Geometry: final body of the model. Coordinates: model frame, mm. Face numbers are marked on the shaded views. A direction names the side the tool comes from. Give positions to 0.01 mm unless a question says otherwise; leave off trailing zeros. Write each loop counter-clockwise with the first axis right and the second up, starting at its lowest first coordinate (ties: lowest second). Pieces come first, ordered by that corner, then holes. Notation, with made-up numbers: M 19,-20 L 29,-20 A11 cw 29,-15 Z; hole C 48,-5 d2. An arc over 180 degrees is marked long. One line per question, with ' | ' between items.
from build123d import *

# Parameters (mm, degrees)
PAD_DEPTH       = 22
SKETCH001_W     = 16
SKETCH001_H     = 16
POCKET_DEPTH    = 39.001
SKETCH002_W     = 38
SKETCH002_H     = 85
POCKET001_DEPTH = 15
SKETCH003_R     = 1.8
POCKET002_DEPTH = 7.001
SKETCH004_R     = 3.6
POCKET003_DEPTH = 3
FILLET_R        = 4
FILLET001_R     = 4
SKETCH005_W     = 87.5
SKETCH005_H     = 3.5
POCKET004_DEPTH = 0.5
SKETCH006_R     = 1.8
POCKET005_DEPTH = 22.001
SKETCH007_R     = 3.6
POCKET006_DEPTH = 3
FILLET002_R     = 4
CHAMFER_SIZE    = 3
SKETCH018_R     = 4.25
POCKET016_DEPTH = 5


with BuildPart() as part:
    # Sketch → Pad (new body)
    with BuildSketch(Plane.XY):
        Polygon((39, 0), (39, 25), (70, 25), (70, 76), (63, 83), (63, 115), (78, 115), (78, 0.241195), align=None)
    extrude(amount=PAD_DEPTH)

    # Sketch001 → Pocket (cut, through all)
    with BuildSketch(Plane.YZ.offset(78)):
        with Locations((7, 15)):
            Rectangle(SKETCH001_W, SKETCH001_H)
        with Locations((108, 15)):
            Rectangle(SKETCH001_W, SKETCH001_H)
    extrude(amount=-POCKET_DEPTH, mode=Mode.SUBTRACT)

    # Sketch002 → Pocket001 (cut)
    with BuildSketch(Plane.XY.offset(22)):
        with Locations((56, 57.5)):
            Rectangle(SKETCH002_W, SKETCH002_H)
    extrude(amount=-POCKET001_DEPTH, mode=Mode.SUBTRACT)

    # Sketch003 → Pocket002 (cut, through all)
    with BuildSketch(Plane.XY.offset(7)):
        with Locations((68, 94.119095)):
            Circle(SKETCH003_R)
        with Locations((44, 20.129047)):
            Circle(SKETCH003_R)
    extrude(amount=-POCKET002_DEPTH, mode=Mode.SUBTRACT)

    # Sketch004 → Pocket003 (cut)
    with BuildSketch(Plane.XY.offset(7)):
        with Locations((68, 94.116013)):
            Circle(SKETCH004_R)
        with Locations((44, 20.124216)):
            Circle(SKETCH004_R)
    extrude(amount=-POCKET003_DEPTH, mode=Mode.SUBTRACT)

    # Fillet
    fillet_edges = [part.edges().sort_by_distance(p)[0] for p in [
        (39, 25, 3.5),
        (70, 25, 3.5),
    ]]
    fillet(fillet_edges, radius=FILLET_R)

    # Fillet001
    fillet001_edges = [part.edges().sort_by_distance(p)[0] for p in [
        (63, 83, 3.5),
        (70, 76, 3.5),
    ]]
    fillet(fillet001_edges, radius=FILLET001_R)

    # Sketch005 → Pocket004 (cut)
    with BuildSketch(Plane.YZ.offset(78)):
        with Locations((57.25, 14.5)):
            Rectangle(SKETCH005_W, SKETCH005_H)
    extrude(amount=-POCKET004_DEPTH, mode=Mode.SUBTRACT)

    # Sketch006 → Pocket005 (cut, through all)
    with BuildSketch(Plane(origin=(0, 0, 0), x_dir=(1, 0, 0), z_dir=(0, 0, -1))):
        with Locations((70, -107.5)):
            Circle(SKETCH006_R)
        with Locations((57.5, -7.5)):
            Circle(SKETCH006_R)
    extrude(amount=-POCKET005_DEPTH, mode=Mode.SUBTRACT)

    # Sketch007 → Pocket006 (cut)
    with BuildSketch(Plane(origin=(0, 0, 0), x_dir=(1, 0, 0), z_dir=(0, 0, -1))):
        with Locations((57.5, -7.5)):
            Circle(SKETCH007_R)
        with Locations((70, -107.5)):
            Circle(SKETCH007_R)
    extrude(amount=-POCKET006_DEPTH, mode=Mode.SUBTRACT)

    # Fillet002
    fillet002_edges = [part.edges().sort_by_distance(p)[0] for p in [
        (39, 0, 3.5),
        (78, 0.241195, 3.5),
        (78, 115, 3.5),
        (63, 115, 3.5),
    ]]
    fillet(fillet002_edges, radius=FILLET002_R)

    # Chamfer
    chamfer_edges = [part.edges().sort_by_distance(p)[0] for p in [
        (75, 57.5, 7),
    ]]
    chamfer(chamfer_edges, length=CHAMFER_SIZE)

    # Sketch018 → Pocket016 (cut, symmetric)
    with BuildSketch(Plane.XY.offset(7)):
        with Locations((44, 20.095486)):
            Circle(SKETCH018_R)
        with Locations((68, 94.107513)):
            Circle(SKETCH018_R)
    extrude(amount=POCKET016_DEPTH, both=True, mode=Mode.SUBTRACT)


solid = part.part
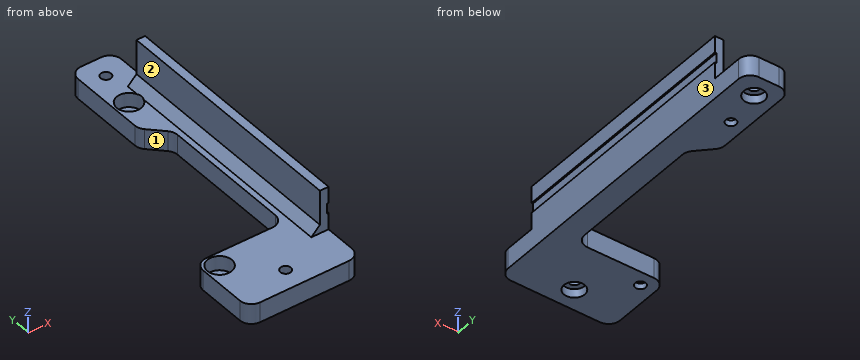
(1) Material intervals for L1, parallel to X at y = 107.5, z = 4.9; L2, parallel to Y at x = 68, z = 1; L3, parallel to Y at x = 44, z = 0.75, sorted ascending. Write a range as [from, to].
Working result:
L1: x = [63, 68.2], [71.8, 78] | L2: y = [0.18, 25.54], [78, 92.32], [95.92, 104.51], [110.49, 115] | L3: y = [0.03, 18.33], [21.93, 25]
(2) Cut plane A-A, the plane y = 7.5. Return loops of the section in (x, z).
Working result:
outline: M 39,0 L 53.9,0 L 53.9,3 L 55.7,3 L 55.7,7 L 39,7 Z; M 59.3,3 L 61.1,3 L 61.1,0 L 78,0 L 78,7 L 59.3,7 Z
(3) Set-up query: the marked faces 1, 2 and 3. Return all of +Z, -Z, +X, -X, +Y, -Y with unobstructed straight access to the full face (end or side cutting, diameter ignored); none if empty.
Working result:
face 1: +Z, -Z, -X | face 2: +Z, -X, +Y, -Y | face 3: +Z, -Z, +X, +Y, -Y
(4) Cut plane C-C, the plane z = 5. Return loops of the section in (x, y).
Working result:
outline: M 39,4.02 A4 ccw 43.02,0.02 L 74.02,0.22 A4 ccw 78,4.22 L 78,111 A4 ccw 74,115 L 67,115 A4 ccw 63,111 L 63,84.66 A4 ccw 64.17,81.83 L 68.83,77.17 A4 cw 70,74.34 L 70,29 A4 cw 66,25 L 43,25 A4 ccw 39,21 Z; hole C 44,20.1 d8.5; hole C 57.5,7.5 d3.6; hole C 68,94.11 d8.5; hole C 70,107.5 d3.6
(5) Cut plane D-D, the plane y = 107.5. Return loops of the section in (x, z).
Working result:
outline: M 63,0 L 66.4,0 L 66.4,3 L 68.2,3 L 68.2,7 L 63,7 Z; M 71.8,3 L 73.6,3 L 73.6,0 L 78,0 L 78,7 L 71.8,7 Z
(6) First-contact query: P1, Ø12, axis at y = 18, z = 17.5, coming from the -X side; P2, Ø9.5, axis at y = 46.5, z = 14, coming from the -X side; P3, Ø7.5, axis at y = 100.5, z = 4, coming from the -X side; P4, Ø8, axis at x = 49, y = 31.5, coming from the -Z side. Flat tips, straight axial feed; report the tip coordinate or a pass-through.
Working result:
P1: stops at x = 75 | P2: stops at x = 74.25 | P3: stops at x = 63 | P4: passes through
(7) Cut plane B-B, the plane y = 60. Return loops of the section in (x, z), then the cut area to 3 significant figures.
Working result:
outline: M 70,0 L 78,0 L 78,12.75 L 77.5,12.75 L 77.5,16.25 L 78,16.25 L 78,22 L 75,22 L 75,10 L 72,7 L 70,7 Z | area: 104 mm^2
